```python
from build123d import *

# Parameters (mm, degrees)
SKETCH1_W           = 15
SKETCH1_H           = 10
BOSS_EXTRUDE1_DEPTH = 1.4
SKETCH2_W           = 15
SKETCH2_H           = 10
SKETCH2_R           = 3.7
BOSS_EXTRUDE2_DEPTH = 3
CUT_EXTRUDE2_DEPTH  = 14.251792332
CHAMFER1_SIZE       = 2.634615696


with BuildPart() as part:
    # Sketch1 → Boss-Extrude1 (new body)
    with BuildSketch(Plane(origin=(0, 0, 0), x_dir=(1, 0, 0), z_dir=(0, 1, 0))):
        Rectangle(SKETCH1_W, SKETCH1_H)
    extrude(amount=BOSS_EXTRUDE1_DEPTH)

    # Sketch2 → Boss-Extrude2 (add)
    with BuildSketch(Plane(origin=(0, 1.4, 0), x_dir=(1, 0, 0), z_dir=(0, 1, 0))):
        Rectangle(SKETCH2_W, SKETCH2_H)
        with Locations(Location((0, 0, 0), (0, 0, 270))):
            Circle(SKETCH2_R, mode=Mode.SUBTRACT)
    extrude(amount=BOSS_EXTRUDE2_DEPTH)

    # Sketch5 → Cut-Extrude2 (cut, through all)
    with BuildSketch(Plane(origin=(0, 0, -5), x_dir=(-1, 0, 0), z_dir=(0, 0, -1))):
        with BuildLine():
            Line((7.5, 0), (-7.5, 0))
            ThreePointArc((-7.5, 0), (0, 0.565700167), (7.5, 0))
        make_face()
    extrude(amount=-CUT_EXTRUDE2_DEPTH, mode=Mode.SUBTRACT)

    # Chamfer1
    # the kernel refuses this chamfer: 3, 2.634615696 mm, written as the material it takes off along each edge
    with BuildSketch(Plane(origin=(7.5, 0, -12.964818141), x_dir=(-0.9928577476807653, 0.11930420307046066, 0), z_dir=(0, 0, 1)), Plane(origin=(-7.5, 0, 12.964818141), x_dir=(0.9928577476807653, 0.1193042030704611, 0), z_dir=(0, 0, -1))) as chamfer1_piece_1:
        with BuildLine():
            Line((3.097426723, 0), (CHAMFER1_SIZE * 0.119304203085, -CHAMFER1_SIZE * 0.992857747804))
            Line((CHAMFER1_SIZE * 0.119304203085, -CHAMFER1_SIZE * 0.992857747804), (0, 0))
            ThreePointArc((0, 0), (1.592490504, -0.023971722), (3.097426723, 0))
        make_face()
    extrude(amount=25.929636281, mode=Mode.SUBTRACT)


solid = part.part
```
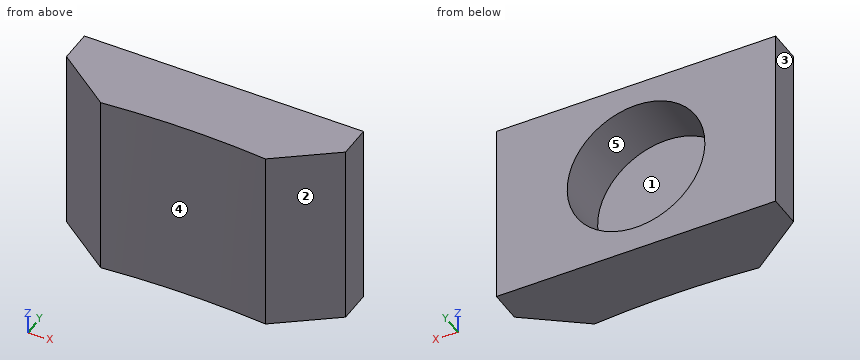
Geometry: final body of the model. Coordinates: model frame, mm. Face numbers are marked on the shaded views. A direction names the side the tool comes from. Round coordinates to 2 decimals unless told otherwise and drop trailing zeros. Order: outer loops, then holes, each group sorted by start corner. A loop starts at its lowest first (then second) coordinate and runs counter-clockwise, first axis right, second up. Notation, with made-up numbers: (44.5, 30) -> (84.5, 30) arc R15 cw to (84.5, 57) -> close; hole circle Ø3 at (2.25, 59.25). An arc over 180 degrees is marked (long way). Write each question's results on one line, items separated by ' | '.
Q1. Pin query (flat end, axial travel): pin 1 Ø6 at (x, z) = (0, 0) entering from +Y; pin 2 Ø1 at (y, z) = (1.5, -3) entering from -X. Return the tip coordinate at first contact, or that it passes through.
Response values:
pin 1: y = 1.4 | pin 2: x = -6.64
Q2. Section query A-A (y = 4.15). Output: boundary loops of the cut face in (x, z), and give its area (3 significant figures).
Response values:
outline: (-7.5, -5) -> (7.5, -5) -> (7.5, 5) -> (-7.5, 5) -> close; hole circle Ø7.4 at (0, 0) | area: 107 mm²
Q3. Pull-direction query (X, two-part tool) for the marked faces 1, 2 and 3; classes: released by +X, released by -X, zero draft, split by the parting line, or undercut.
Response values:
face 1: undercut | face 2: released by +X | face 3: released by -X
Q4. Ray query, line 1 along X through (y, z) = (3.2, 0); line 2 along Y through (x, z) = (-0.25, -2.5); line 3 along X through (y, z) = (2, 0). Return the intervals inside material, ascending.
Response values:
line 1: -7.5 to -3.7, 3.7 to 7.5 | line 2: 0.57 to 1.4 | line 3: -6.64 to -3.7, 3.7 to 6.64
Q5. Section query B-B (z = 0). Output: boundary loops of the cut face in (x, y).
Response values:
outline: (-7.5, 2.63) -> (-4.42, 0.37) arc R50 cw to (4.42, 0.37) -> (7.5, 2.63) -> (7.5, 4.4) -> (3.7, 4.4) -> (3.7, 1.4) -> (-3.7, 1.4) -> (-3.7, 4.4) -> (-7.5, 4.4) -> close
Q6. Section query D-D (y = 1.6). Output: boundary loops of the cut face in (x, z), and give its area (3 significant figures).
Response values:
outline: (-6.1, -5) -> (6.1, -5) -> (6.1, 5) -> (-6.1, 5) -> close; hole circle Ø7.4 at (0, 0) | area: 78.9 mm²
Q7. Access query for the marked faces 4 and 5. Directions: +Z, -Z, +X, -X, +Y, -Y. A direction counts if a zero-diameter tool reaches every point of the face in a straight line with its end or side. Return the directions, or none.
Response values:
face 4: +Z, -Z, -Y | face 5: +Y
Q8. Section query C-C (x = 0). Output: boundary loops of the cut face in (y, z), and give its area (3 significant figures).
Response values:
outline: (0.57, -5) -> (4.4, -5) -> (4.4, -3.7) -> (1.4, -3.7) -> (1.4, 3.7) -> (4.4, 3.7) -> (4.4, 5) -> (0.57, 5) -> close | area: 16.1 mm²
